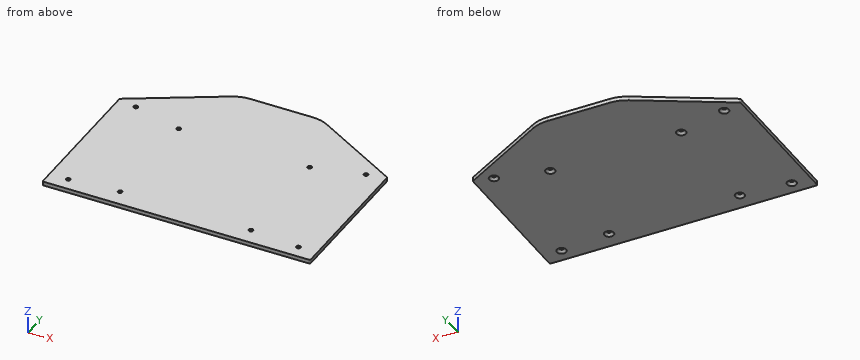
Solid Edge part; units mm, degrees
sketch "Sketch1" plane through (0, 0, -20) normal (0, 0, -1) x (-1, 0, 0)
  line L0 (-99.4961, 55.2879) -> (-35.7644, 91.7061)
  arc A0 (-35.7644, 91.7061) -> (-23.3609, 95) centre (-23.3609, 70) cw
  line L1 (-23.3609, 95) -> (-19.45, 95)
  line L2 (-19.45, 95) -> (-13.95, 95)
  line L3 (-13.95, 95) -> (23.3609, 95)
  arc A1 (23.3609, 95) -> (35.7644, 91.7061) centre (23.3609, 70) cw
  line L4 (35.7644, 91.7061) -> (99.4961, 55.2879)
  arc A2 (99.4961, 55.2879) -> (100, 54.4197) centre (99, 54.4197) cw
  line L5 (100, 54.4197) -> (100, -54)
  arc A3 (100, -54) -> (99, -55) centre (99, -54) cw
  line L6 (99, -55) -> (-99, -55)
  arc A4 (-99, -55) -> (-100, -54) centre (-99, -54) cw
  line L7 (-100, -54) -> (-100, 54.4197)
  arc A5 (-100, 54.4197) -> (-99.4961, 55.2879) centre (-99, 54.4197) cw
extrude "Extrusionsausprägung_1" add sketch "Sketch1" along normal blind 3
hole "Bohrung_1" at (86, 51.4825, -23) direction (0, 0, 1) diameter 3.2 end through all countersink diameter 6.94 countersink angle 90
hole "Hole1" at (86, -45, -23) direction (0, 0, 1) diameter 3.2 end through all countersink diameter 6.94 countersink angle 90
hole "Hole2" at (-86, 51.4825, -23) direction (0, 0, 1) diameter 3.2 end through all countersink diameter 6.94 countersink angle 90
hole "Hole3" at (-86, -45, -23) direction (0, 0, 1) diameter 3.2 end through all countersink diameter 6.94 countersink angle 90
hole "Hole4" at (48.895, 41.91, -23) direction (0, 0, 1) diameter 3.2 end through all countersink diameter 6.94 countersink angle 90
hole "Hole5" at (-48.895, 41.91, -23) direction (0, 0, 1) diameter 3.2 end through all countersink diameter 6.94 countersink angle 90
hole "Hole6" at (-48.895, -41.91, -23) direction (0, 0, 1) diameter 3.2 end through all countersink diameter 6.94 countersink angle 90
hole "Hole7" at (48.895, -41.91, -23) direction (0, 0, 1) diameter 3.2 end through all countersink diameter 6.94 countersink angle 90
Could you check a few things on this model? Use its own coordinates, in mm. Coordinates: 2 decimals unless noted, no trailing zeros. Order: outer loops, then holes, each group sorted by start corner. A loop starts at its lowest first (then second) coordinate and runs counter-clockwise, first axis right, second up. Notation, with made-up numbers: (43.25, 44) -> (58.25, 44) arc R17 cw to (58.25, 53) -> close; hole circle Ø1 at (-3.75, 48.5). An arc over 180 degrees is marked (long way). One line per item, written item: value. Start each with the question number.
1) I'm going to push flat-ended pins straight in: pin 1 (4 mm diameter, centred on x = 48.895, y = 41.91, fed in from -Z); pin 2 (1.5 mm diameter, centred on y = 61.5, z = -21, fed in from -X); pin 3 (3.5 mm diameter, centred on x = -48.895, y = -41.91, fed in from -Z). Where does each tip first touch, or does it pass through?
2) Imagine slicing it at B-B on x = 55. List the corners of the cut face in (y, z) for me, plus the area to 3 significant figures.
3) If I drill on L1, parallel to X at y = 41.91, z = -20.35 (3 decimals); L2, parallel to Y at x = -86, z = -20.25; L3, parallel to X at y = 51, z = -20.9, over which ranges is the centre line in solid material (lowest first)? Write a range as [from, to].
4) Imagine slicing it at A-A on z = -21.65. Count the separate pieces of the cut face and the enclosed holes in it, plus the area to 3 significant figures.
5) Imagine slicing it at C-C on x = -80.5. List the corners of the cut face in (y, z) for me, plus the area to 3 significant figures.
Answer list:
1. pin 1: stops at z = -21.53
1. pin 2: stops at x = -89.94
1. pin 3: stops at z = -21.28
2. outline: (-55, -23) -> (80.71, -23) -> (80.71, -20) -> (-55, -20) -> close
2. area: 407 mm2
3. L1: x = [-100, -50.495], [-47.295, 47.295], [50.495, 100]
3. L2: y = [-55, -46.6], [-43.4, 49.88], [53.08, 63]
3. L3: x = [-100, -87.53], [-84.47, 84.47], [87.53, 100]
4. separate pieces: 1
4. enclosed holes: 8
4. area: 27,100 mm2
5. outline: (-55, -23) -> (66.14, -23) -> (66.14, -20) -> (-55, -20) -> close
5. area: 363 mm2
